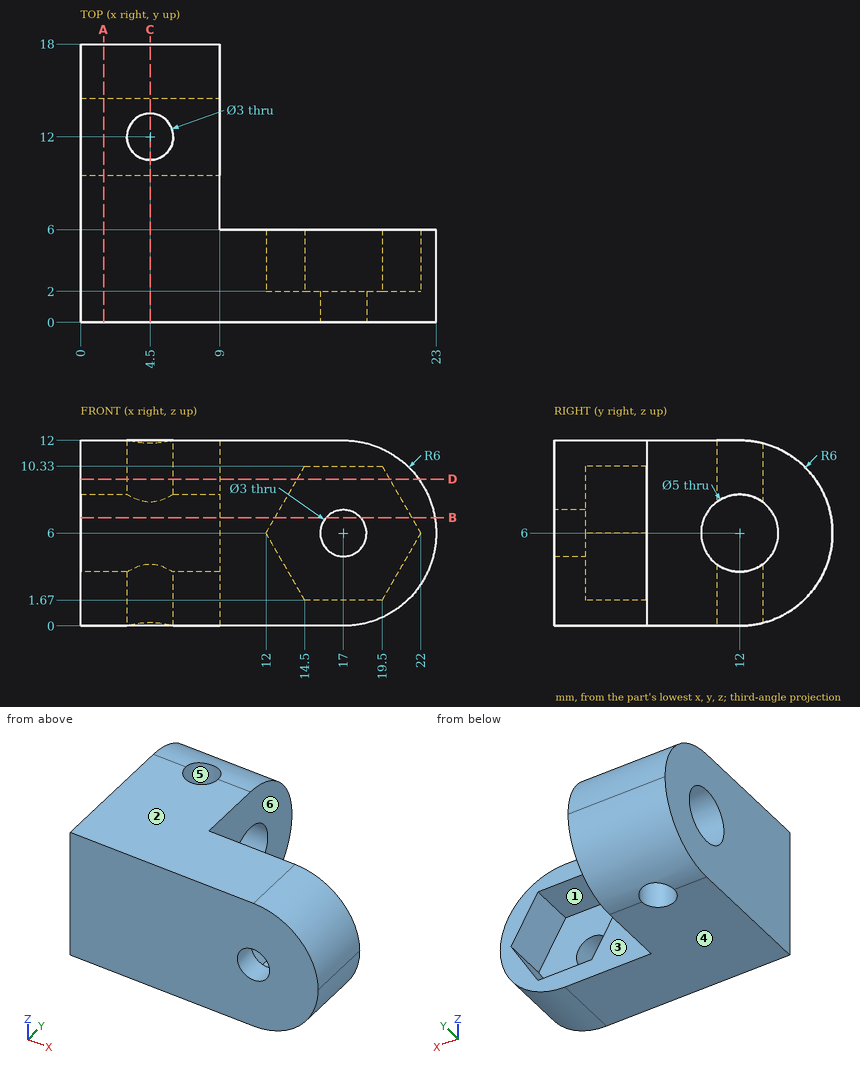
Verification items for this drawing (mm, ordinates from the low corner). A direction names the side the tool comes from. Round coordinates to 2 decimals unless told otherwise and drop trailing zeros. Write each loop counter-clockwise with the first axis right and the second up, starting at its lowest first coordinate (ties: lowest second). Pieces come first, ordered by that corner, then holes. Notation, with made-up numbers: (24.25, 34.5) - (34.25, 34.5) arc R16 cw to (34.25, 52.5) - close; hole circle Ø9 at (38.25, 78.25). An arc over 180 degrees is marked (long way). Answer as a JSON object with one key per item and string values. Group by question number.
Q1. Section check B-B, the plane z = 7. Enter the section's corners in (x, y), plus the area to 3 significant figures.
Q2. Go/stop test with flat-tipped pins: pin 1 Ø3.5 at (y, z) = (15, 6.5) entering from +X; pin 2 Ø1 at (x, z) = (20, 2.5) entering from +Y. Record where each tip stops, or that it passes through.
Q3. Section check A-A, the plane x = 1.5. Enter the section's corners in (y, z), plus the area to 3 significant figures.
Q4. Thickness scan on line 1 (Z direction, x = 16.25, y = 4); line 2 (X direction, y = 12, z = 1.1); line 3 (X direction, y = 7.25, z = 4.75). Record the ranges inside material, lowest first.
Q5. Tool access check on the marked faces 1, 2 and 3. Record the directions out of +Z, -Z, +X, -X, +Y, -Y that give a thin tool (end or side, any length) a straight path to the whole face; none if there is none.
Q6. Section check C-C, the plane x = 4.5. Enter the section's corners in (y, z).
Q7. Mould release check, pull along X, two halves, no side actions. Record for the marked faces 4, 5 and 6: released by +X, released by -X, zero draft, split by the parting line, or undercut.
Q8. Section check D-D, the plane z = 9.5. Enter the section's corners in (x, y), plus the area to 3 significant figures.
Found:
{
 "1": {"outline": "(0, 0) - (15.88, 0) - (15.88, 2) - (12.58, 2) - (12.58, 6) - (9, 6) - (9, 9.71) - (0, 9.71) - close; (0, 14.29) - (9, 14.29) - (9, 17.92) - (0, 17.92) - close; (18.12, 0) - (22.92, 0) - (22.92, 6) - (21.42, 6) - (21.42, 2) - (18.12, 2) - close", "area": "164 mm^2"},
 "2": {"pin 1": "stops at x = 9", "pin 2": "stops at y = 6"},
 "3": {"outline": "(0, 0) - (12, 0) arc R6 ccw to (12, 12) - (0, 12) - close; hole circle Ø5 at (12, 6)", "area": "181 mm^2"},
 "4": {"line 1": "z = 0 to 1.67, 10.33 to 12", "line 2": "x = 0 to 3, 6 to 9", "line 3": "x = 0 to 9"},
 "5": {"face 1": "+Y", "face 2": "+Z, +X, -X, +Y, -Y", "face 3": "+Z, -Z, +X, +Y"},
 "6": {"outline": "(0, 0) - (10.5, 0) - (10.5, 4) arc R2.5 cw to (10.5, 8) - (10.5, 12) - (0, 12) - close; (13.5, 0.19) arc R6 ccw to (13.5, 11.81) - (13.5, 8) arc R2.5 cw to (13.5, 4) - close"},
 "7": {"face 4": "zero draft", "face 5": "undercut", "face 6": "released by +X"},
 "8": {"outline": "(0, 0) - (21.87, 0) - (21.87, 6) - (19.98, 6) - (19.98, 2) - (14.02, 2) - (14.02, 6) - (9, 6) - (9, 16.87) - (0, 16.87) - close; hole circle Ø3 at (4.5, 12)", "area": "198 mm^2"}
}
